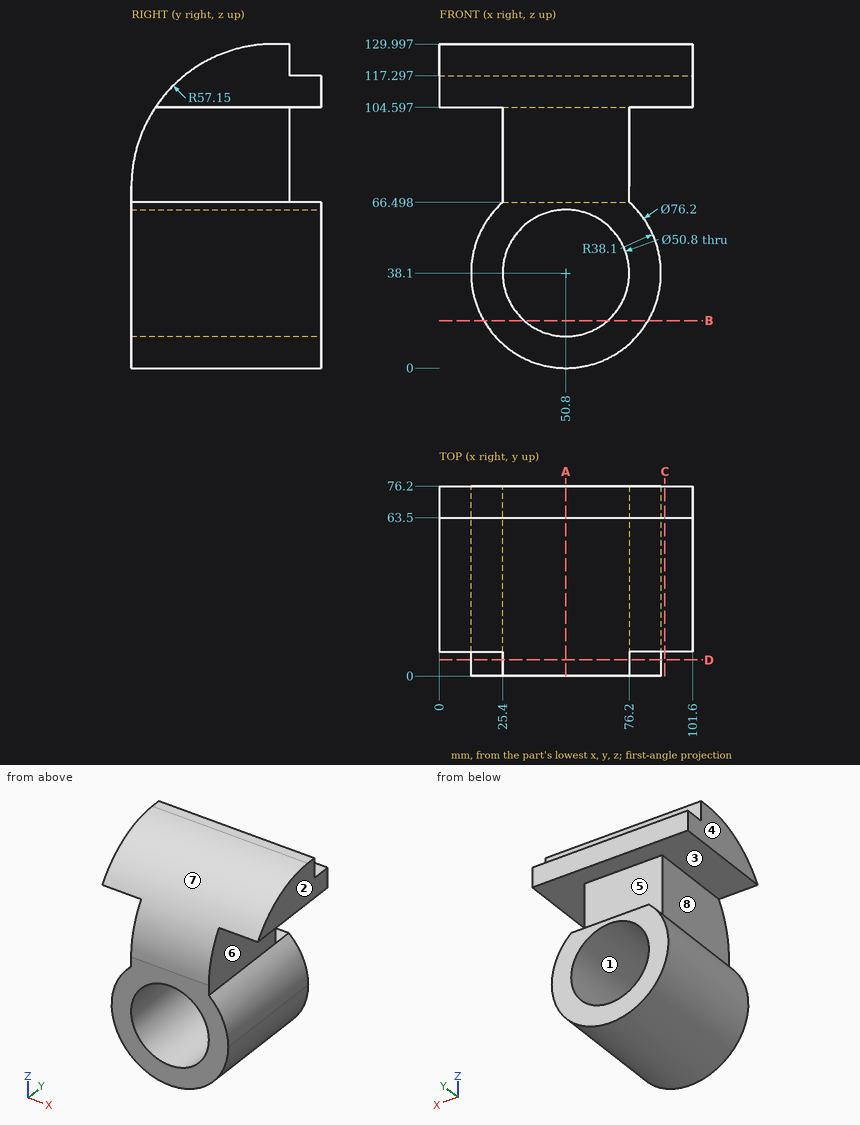
Source: three-view drawing plus pictorial views. Frame: mm from the lowest corner of the part. A direction names the side the tool comes from. Give positions to 0.01 mm unless a question says otherwise; leave off trailing zeros. Order: outer loops, then holes, each group sorted by start corner. A loop starts at its lowest first (then second) coordinate and runs counter-clockwise, first axis right, second up. Notation, with made-up numbers: M 2.5,74 L 51.5,74 A16 ccw 51.5,102 Z; hole C 50.25,-10 d2. An arc over 180 degrees is marked long. Return JSON: item names as keys, results as strings.
1) Section query A-A on x = 50.8. Output: boundary loops of the cut face in (y, z).
Taken from the geometry:
{"outline": "M 0,0 L 76.2,0 L 76.2,12.7 L 0,12.7 Z; M 0,63.5 L 76.2,63.5 L 76.2,66.5 L 63.5,66.5 L 63.5,104.6 L 76.2,104.6 L 76.2,117.3 L 63.5,117.3 L 63.5,130 L 57.15,130 A57.15 ccw 0,72.85 Z"}
2) Access query for the marked faces 5, 6, 7 and 8. Directions: +Z, -Z, +X, -X, +Y, -Y. A direction counts if a zero-diameter tool reaches every point of the face in a straight line with its end or side. Return the directions, or none.
Taken from the geometry:
{"face 5": "+X, -X, +Y", "face 6": "+X, +Y, -Y", "face 7": "+Z, +X, -X, -Y", "face 8": "-X, +Y, -Y"}
3) Section query B-B on z = 19. Output: boundary loops of the cut face in (x, y), and give its area (3 significant figures).
Taken from the geometry:
{"outline": "M 17.83,0 L 34.06,0 L 34.06,76.2 L 17.83,76.2 Z; M 67.54,0 L 83.77,0 L 83.77,76.2 L 67.54,76.2 Z", "area": "2,470 mm2"}
4) Line query: L1, parallel to Z at x = 50, y = 59; L2, parallel to X at y = 45, z = 38; L3, parallel to X at y = 34.5, z = 43. Output: solid intervals per line, ascending. Write a range as [from, to].
Taken from the geometry:
{"L1": "z = [0.01, 12.71], [63.49, 130]", "L2": "x = [12.7, 25.4], [76.2, 88.9]", "L3": "x = [13.02, 25.88], [75.72, 88.58]"}
5) Contact query for flat-ended pins moving along their axis: pin 1 (4 mm diameter, centred on x = 40, y = 40, fed in from -Z); pin 2 (1 mm diameter, centred on x = 46, y = 18, fed in from +Z); pin 3 (10 mm diameter, centred on x = 45, z = 93, fed in from -Y). Output: stop coordinate, or through.
Taken from the geometry:
{"pin 1": "stops at z = 1.03", "pin 2": "stops at z = 114.95", "pin 3": "stops at y = 2.05"}
6) Mould query, pull axis X, two halves, no side actions, for the marked faces 1, 2, 3 and 4. Classes: released by +X, released by -X, zero draft, split by the parting line, or undercut.
Taken from the geometry:
{"face 1": "undercut", "face 2": "released by +X", "face 3": "zero draft", "face 4": "released by -X"}
7) Section query C-C on x = 90.5. Output: boundary loops of the cut face in (y, z), and give its area (3 significant figures).
Taken from the geometry:
{"outline": "M 9.63,104.6 L 76.2,104.6 L 76.2,117.3 L 63.5,117.3 L 63.5,130 L 57.15,130 A57.15 ccw Z", "area": "1,170 mm2"}
8) Section query D-D on y = 6.5. Output: boundary loops of the cut face in (x, z).
Taken from the geometry:
{"outline": "M 25.4,66.5 A38.1 ccw long 76.2,66.5 L 76.2,99.32 L 25.4,99.32 Z; hole C 50.8,38.1 d50.8"}
